For this review, use the dimensioned drawing (mm, ordinates from the lowest corner) and the shaded views. A direction names the side the tool comes from. Round coordinates to 2 decimals unless told otherwise and drop trailing zeros. Loops run counter-clockwise (first coordinate to the right, second up) from the corner with the lowest first, then second, coordinate; pieces in that order, holes last. Notation, with made-up numbers: M -24,-37.5 L 20,-37.5 A19 cw 20,-20.5 Z; hole C 35,-1 d11. An arc over 180 degrees is marked long. One line per item, written item: value. Start each with the question number.
Item 1: Mouldability with a two-part tool opening along X and no side actions: class the marked faces 1, 2, 3 and 4 as released by +X, released by -X, zero draft, split by the parting line, or undercut.
Item 2: We need section C-C (z = 71). Write out the cut boundary in (x, y).
Item 3: Clearance check with flat-ended pins moving along their axes: pin 1 (2 mm diameter, centred on y = 19, z = 48.5, fed in from -X); pin 2 (1 mm diameter, centred on y = 8.5, z = 35.5, fed in from -X) (1 decimal); pin 3 (12 mm diameter, centred on y = 20, z = 38, fed in from -X). State where each tip first meets the part, or that it passes through.
Item 4: We need section A-A (z = 57.5). Write out the cut boundary in (x, y), then the cut area to 3 significant figures.
Item 5: We need section D-D (x = 18). Write out the cut boundary in (y, z).
Item 6: For line 1 along X through (y, z) = (10.75, 65.5); line 2 along X through (y, z) = (13.75, 34) (1 decimal); line 3 along Z through (x, y) = (98.5, 2.75) (1 decimal), list the stretches that pass through material, from the lowest coordinate up.
Item 7: For the marked faces 5 and 6, list the 3-axis set-ups (+Z, -Z, +X, -X, +Y, -Y) from which the entire face can be reached by the end or side of a thin tool; tool diameter is ignored.
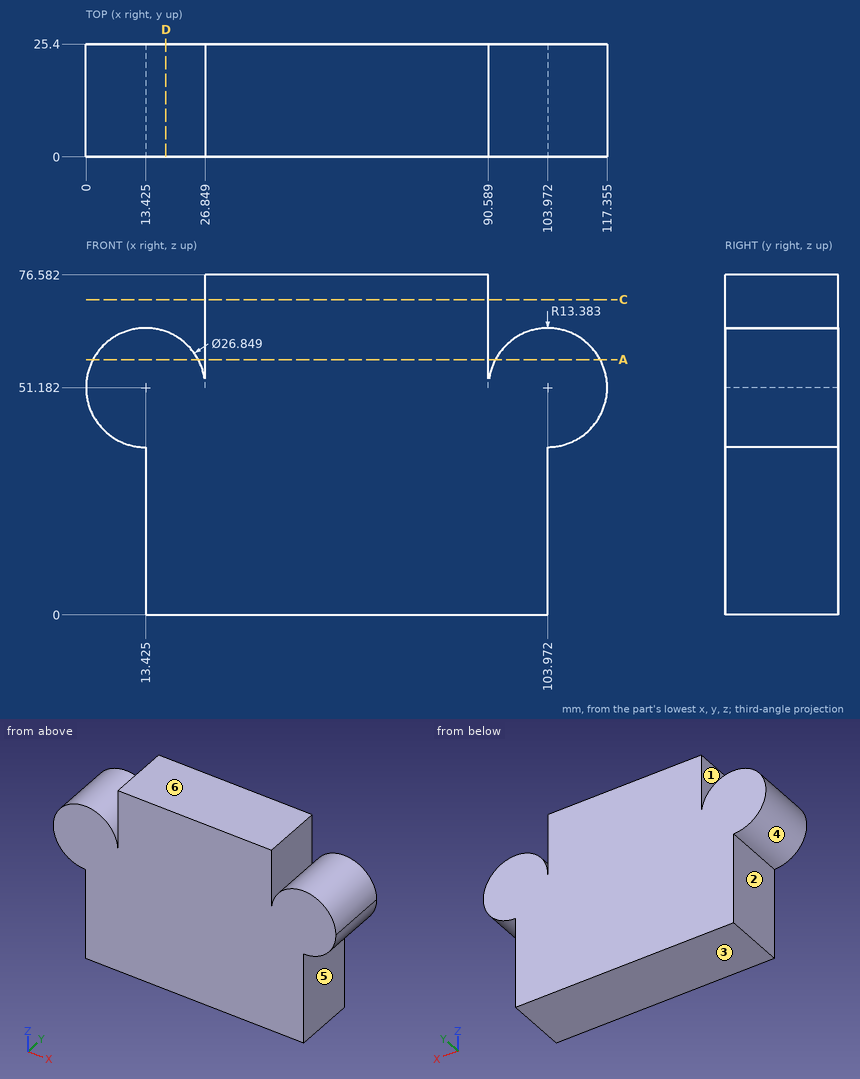
A:
1. face 1: undercut
1. face 2: released by -X
1. face 3: zero draft
1. face 4: undercut
2. outline: M 26.85,0 L 90.59,0 L 90.59,25.4 L 26.85,25.4 Z
3. pin 1: x = 0.11
3. pin 2: x = 13.4
3. pin 3: x = 2.08
4. outline: M 1.58,0 L 25.27,0 L 25.27,25.4 L 1.58,25.4 Z; M 26.85,0 L 90.59,0 L 90.59,25.4 L 26.85,25.4 Z; M 92.17,0 L 115.77,0 L 115.77,25.4 L 92.17,25.4 Z
4. area: 2,820 mm2
5. outline: M 0,0 L 25.4,0 L 25.4,63.8 L 0,63.8 Z
6. line 1: 26.85 to 90.59
6. line 2: 13.4 to 104
6. line 3: 0 to 63.4
7. face 5: -Z, +X, +Y, -Y
7. face 6: +Z, +X, -X, +Y, -Y
